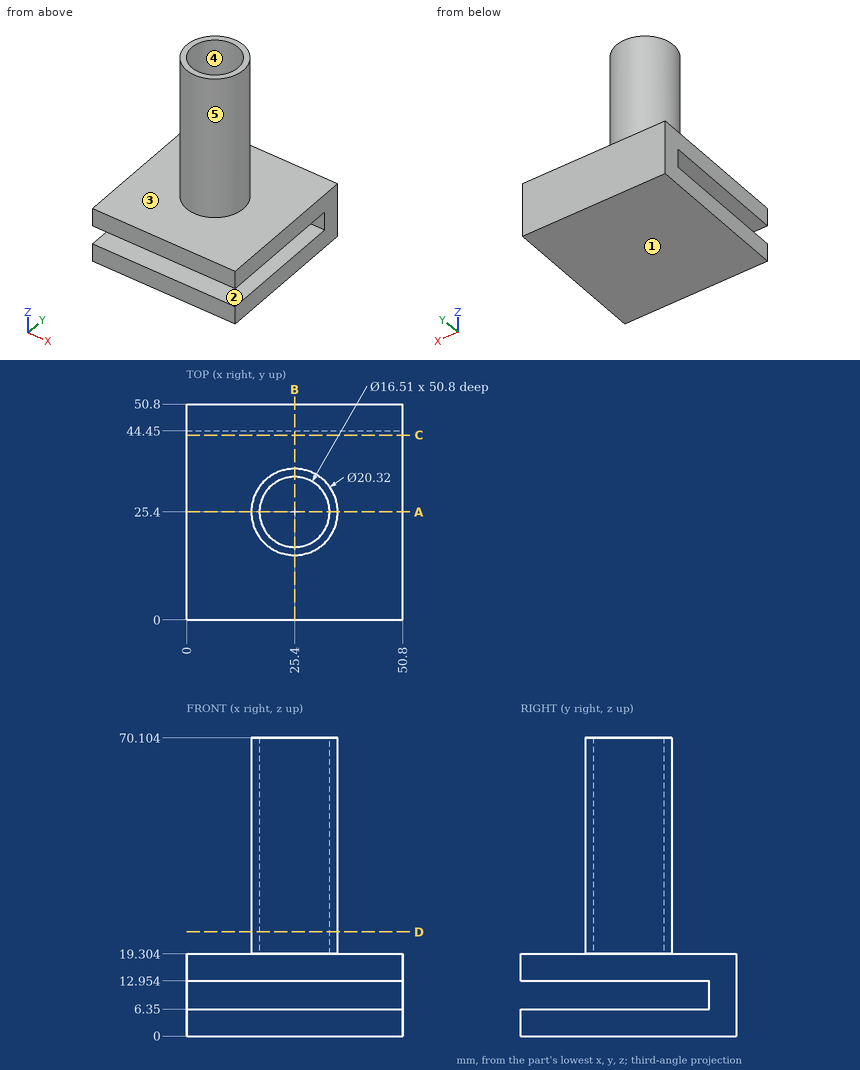
Geometry: see drawing. Coordinates: mm, zero at the bounding-box minimum. A direction names the side the tool comes from. Round coordinates to 2 decimals unless told otherwise and drop trailing zeros. Order: outer loops, then holes, each group sorted by start corner. A loop starts at its lowest first (then second) coordinate and runs counter-clockwise, first axis right, second up. Notation, with made-up numbers: (72, 41) - (105, 41) arc R12 ccw to (105, 59) - close; hole circle Ø3 at (41, 89). An arc over 180 degrees is marked (long way). Use a Markdown table: item, result. Add a question column.
1. Set-up query: the marked faces 1 and 2. Return all of +Z, -Z, +X, -X, +Y, -Y with unobstructed straight access to the full face (end or side cutting, diameter ignored); none if empty.
2. Mould query, pull axis Y, two halves, no side actions, for the marked faces 3, 4 and 5. Classes: +Y half, -Y half, draft (parallel to the pull), parting line (faces both ways), or undercut.
3. Line query: probe 1 along Z at (x, y) = (28.5, 23.5); probe 2 along Y at (x, z) = (25, 33); probe 3 along Z at (x, y) = (35.5, 25.5). Output: solid intervals per line, ascending.
4. Section query C-C (y = 43.5). Return the cut outline in (x, z).
5. First-contact query: pin 1 (8 mm diameter, centred on x = 25.5, z = 30, fed in from +Y); pin 2 (1 mm diameter, centred on x = 38, y = 22.5, fed in from +Z); pin 3 (6 mm diameter, centred on y = 26.5, z = 23.5, fed in from +X). Flat tips, straight axial feed; report the tip coordinate or a pass-through.
6. Section query A-A (y = 25.4). Return the cut outline in (x, z) (3 decimals).
7. Section query D-D (z = 24.5). Return the cut outline in (x, y) (3 decimals).
8. Section query B-B (x = 25.4). Return the cut outline in (y, z) (3 decimals), then the cut area to 3 significant figures.
Derived:
| question | item | result |
|---|---|---|
| 1 | face 1 | -Z, +X, -X, +Y, -Y |
| 1 | face 2 | +X, -X, -Y |
| 2 | face 3 | draft |
| 2 | face 4 | undercut |
| 2 | face 5 | parting line |
| 3 | probe 1 | 0 to 6.35, 12.95 to 19.3 |
| 3 | probe 2 | 15.25 to 17.15, 33.65 to 35.55 |
| 3 | probe 3 | 0 to 6.35, 12.95 to 70.1 |
| 4 | outline | (0, 0) - (50.8, 0) - (50.8, 6.35) - (0, 6.35) - close; (0, 12.95) - (50.8, 12.95) - (50.8, 19.3) - (0, 19.3) - close |
| 5 | pin 1 | y = 35.56 |
| 5 | pin 2 | z = 19.3 |
| 5 | pin 3 | x = 35.56 |
| 6 | outline | (0, 0) - (50.8, 0) - (50.8, 6.35) - (0, 6.35) - close; (0, 12.954) - (50.8, 12.954) - (50.8, 19.304) - (35.56, 19.304) - (35.56, 70.104) - (33.655, 70.104) - (33.655, 19.304) - (17.145, 19.304) - (17.145, 70.104) - (15.24, 70.104) - (15.24, 19.304) - (0, 19.304) - close |
| 7 | outline | circle Ø20.32 at (25.4, 25.4); hole circle Ø16.51 at (25.4, 25.4) |
| 8 | outline | (0, 0) - (50.8, 0) - (50.8, 19.304) - (35.56, 19.304) - (35.56, 70.104) - (33.655, 70.104) - (33.655, 19.304) - (17.145, 19.304) - (17.145, 70.104) - (15.24, 70.104) - (15.24, 19.304) - (0, 19.304) - (0, 12.954) - (44.45, 12.954) - (44.45, 6.35) - (0, 6.35) - close |
| 8 | area | 881 mm2 |
